Design review of the part built by this model. Coordinates are the model's own, in mm. A direction names the side the tool comes from. Coordinates: 2 decimals unless noted, no trailing zeros. Write each loop counter-clockwise with the first axis right and the second up, starting at its lowest first coordinate (ties: lowest second). Pieces come first, ordered by that corner, then holes. Notation, with made-up numbers: (-31, -1.5) - (-13, -1.5) arc R11 cw to (-13, 2.5) - close; hole circle Ø10 at (-24, -20.75). An arc over 180 degrees is marked (long way). Answer as CSV lines item,"result". Start each with the question number.
Q1. We need section A-A (x = -0.5). Write out the cut boundary in (y, z).
Q2. Mouldability with a two-part tool opening along Y and no side actions: class faces 4 (the face through (4.19, -5.25, 9.86)), 5 (the face through (10, 7, 10)), 6 (the face through (2, -3.9, 10)), 7 (the face through (-2, 3.9, 10)) as pulls with the +Y half, pulls with the -Y half, needs draft (parallel to the pull), parting line crosses it, or undercut.
Q3. We need section B-B (y = 5). Write out the cut boundary in (x, z), plus the area to 3 significant figures.
Q4. For line 1 along Y through (x, z) = (-7, 12.25); line 2 along X through (y, z) = (4.5, 12), list the stretches that pass through material, from the lowest coordinate up. Write a range as [from, to].
Q5. Clearance check with flat-ended pins moving along their axes: pin 1 (12 mm diameter, centred on x = -3, z = 4.5, fed in from -Y); pin 2 (4 mm diameter, centred on y = 0, z = 9.5, fed in from +X); pin 3 (3 mm diameter, centred on y = 2, z = 11.5, fed in from +X); pin 4 (2 mm diameter, centred on x = 2, z = 6.5, fed in from +Y). State where each tip first meets the part, or that it passes through.
Q6. Machinability: for faces 1 (the face through (-3.9, 2, 10)), 2 (the face through (3.9, -2, 10)), 3 (the face through (-5.21, 4.15, 9.86)), which of the approach directions +Z, -Z, +X, -X, +Y, -Y give a long, thin tool a straight path to every point of the face, cutting with its end or side? Answer none if there is none.
Q7. We need section C-C (y = -1.5). Write out the cut boundary in (x, z).
Q8. We need section D-D (y = -4.25). Write out the cut boundary in (x, z).
from build123d import *

# Parameters (mm, degrees)
BOSS_EXTRU_1_DEPTH           = 20
R_P_TITION_CIRCULAIRE1_COUNT = 4


with BuildPart() as part:
    # Esquisse1 → Boss.-Extru.1 (new body)
    with BuildSketch(Plane.XY):
        with BuildLine():
            Line((-9.5, 10), (-4.58, 10))
            Line((-4.58, 10), (-3.125, 8.545))
            Line((-3.125, 8.545), (-3.125, 8.2))
            Line((-3.125, 8.2), (-5.5, 8.2))
            Line((-5.5, 8.2), (-5.5, 6.560660172))
            Line((-5.5, 6.560660172), (-2.839339828, 3.9))
            Line((-2.839339828, 3.9), (-0.21, 3.9))
            Line((-0.21, 3.9), (0, 3.69))
            Line((0, 3.69), (0, 2.1))
            ThreePointArc((0, 2.1), (-1.48492424, 1.48492424), (-2.1, 0))
            Line((-2.1, 0), (-3.69, 0))
            Line((-3.69, 0), (-3.9, 0.21))
            Line((-3.9, 0.21), (-3.9, 2.839339828))
            Line((-3.9, 2.839339828), (-6.560660172, 5.5))
            Line((-6.560660172, 5.5), (-8.2, 5.5))
            Line((-8.2, 5.5), (-8.2, 3.125))
            Line((-8.2, 3.125), (-8.545, 3.125))
            Line((-8.545, 3.125), (-10, 4.58))
            Line((-10, 4.58), (-10, 9.5))
            ThreePointArc((-10, 9.5), (-9.853553391, 9.853553391), (-9.5, 10))
        make_face()
    boss_extru_1 = extrude(amount=BOSS_EXTRU_1_DEPTH)

    # R_p_tition circulaire1: Boss.-Extru.1 ×4 about axis
    r_p_tition_circulaire1_axis = Axis((0, 0, 0), (0, 0, 1))
    for i in range(1, R_P_TITION_CIRCULAIRE1_COUNT):
        add(boss_extru_1.rotate(r_p_tition_circulaire1_axis, i * 360 / R_P_TITION_CIRCULAIRE1_COUNT))


solid = part.part
Results list:
1,outline,"(-3.9, 0) - (-2.04, 0) - (-2.04, 20) - (-3.9, 20) - close; (2.04, 0) - (3.9, 0) - (3.9, 20) - (2.04, 20) - close"
2,face 4,"undercut"
2,face 5,"needs draft"
2,face 6,"pulls with the -Y half"
2,face 7,"pulls with the +Y half"
3,outline,"(-10, 0) - (-8.2, 0) - (-8.2, 20) - (-10, 20) - close; (-6.06, 0) - (-3.94, 0) - (-3.94, 20) - (-6.06, 20) - close; (3.94, 0) - (6.06, 0) - (6.06, 20) - (3.94, 20) - close; (8.2, 0) - (10, 0) - (10, 20) - (8.2, 20) - close"
3,area,"157 mm2"
4,line 1,"y = [-10, -5.5], [5.5, 10]"
4,line 2,"x = [-9.92, -8.2], [-5.56, -3.44], [3.44, 5.56], [8.2, 9.92]"
5,pin 1,"stops at y = -10"
5,pin 2,"stops at x = 3.9"
5,pin 3,"stops at x = 8.92"
5,pin 4,"stops at y = 4.06"
6,face 1,"+Z, -Z, -X"
6,face 2,"+Z, -Z, +X"
6,face 3,"+Z, -Z"
7,outline,"(-3.9, 0) - (-1.47, 0) - (-1.47, 20) - (-3.9, 20) - close; (1.47, 0) - (3.9, 0) - (3.9, 20) - (1.47, 20) - close"
8,outline,"(-9.67, 0) - (-8.2, 0) - (-8.2, 20) - (-9.67, 20) - close; (-5.31, 0) - (-3.19, 0) - (-3.19, 20) - (-5.31, 20) - close; (3.19, 0) - (5.31, 0) - (5.31, 20) - (3.19, 20) - close; (8.2, 0) - (9.67, 0) - (9.67, 20) - (8.2, 20) - close"
